Read the model definition and answer for the solid it produces. Units are mm, in the model's axes. Round coordinates to 2 decimals unless told otherwise and drop trailing zeros. Use a Markdown table: item, result. Add a question column.
1. The mould has two halves that part along X. Classify faces 1 (the face through (96, 0.5, -2)), 2 (the face through (52.3, 0.2, 13.6)), 3 (the face through (42.69, 0.25, -6.85)): +X half, -X half, draft (parallel to the pull), parting line (faces both ways), or undercut.
2. Section A-A, the plane y = 0.35 is taken. Give the number of separate pieces and of enclosed holes in the cut face, then the cut area to 3 significant figures.
3. Consider L1, parallel to Z at x = 58, y = 0.4; L2, parallel to Z at x = 27, y = 0.2. Determine where each line is inside the solid, lowest interval first. Write a range as [from, to].
```python
from build123d import *

# Parameters (mm, degrees)
SKETCH1_W           = 192.336493245
SKETCH1_H           = 38.107536872
BOSS_EXTRUDE1_DEPTH = 0.5


with BuildPart() as part:
    # Sketch1 → Boss-Extrude1 (new body)
    with BuildSketch(Plane(origin=(0, 0, 0), x_dir=(1, 0, 0), z_dir=(0, 1, 0))):
        with Locations((76.086163536, 1.75)):
            Rectangle(SKETCH1_W, SKETCH1_H)
        with BuildLine():
            Line((-17.791271396, 9.694580127), (-8.803798051, 0.707106781))
            ThreePointArc((-8.803798051, 0.707106781), (-7.096691269, 0), (-8.803798051, -0.707106781))
            Line((-8.803798051, -0.707106781), (-17.791271396, -9.694580127))
            ThreePointArc((-17.791271396, -9.694580127), (-17.791271396, -13.512956745), (-13.972894778, -13.512956745))
            Line((-13.972894778, -13.512956745), (-0.459938033, 0))
            Line((-0.459938033, 0), (-13.972894778, 13.512956745))
            ThreePointArc((-13.972894778, 13.512956745), (-17.791271396, 13.512956745), (-17.791271396, 9.694580127))
        make_face(mode=Mode.SUBTRACT)
        with BuildLine():
            Line((-3.972894778, 13.512956745), (9.540061967, 0))
            Line((9.540061967, 0), (-3.972894778, -13.512956745))
            ThreePointArc((-3.972894778, -13.512956745), (-7.791271396, -13.512956745), (-7.791271396, -9.694580127))
            Line((-7.791271396, -9.694580127), (1.196201949, -0.707106781))
            ThreePointArc((1.196201949, -0.707106781), (2.903308731, 0), (1.196201949, 0.707106781))
            Line((1.196201949, 0.707106781), (-7.791271396, 9.694580127))
            ThreePointArc((-7.791271396, 9.694580127), (-7.791271396, 13.512956745), (-3.972894778, 13.512956745))
        make_face(mode=Mode.SUBTRACT)
        with BuildLine():
            Line((6.027105222, 13.512956745), (19.540061967, 0))
            Line((19.540061967, 0), (6.027105222, -13.512956745))
            ThreePointArc((6.027105222, -13.512956745), (2.208728604, -13.512956745), (2.208728604, -9.694580127))
            Line((2.208728604, -9.694580127), (11.196201949, -0.707106781))
            ThreePointArc((11.196201949, -0.707106781), (12.903308731, 0), (11.196201949, 0.707106781))
            Line((11.196201949, 0.707106781), (2.208728604, 9.694580127))
            ThreePointArc((2.208728604, 9.694580127), (2.208728604, 13.512956745), (6.027105222, 13.512956745))
        make_face(mode=Mode.SUBTRACT)
        with BuildLine():
            Line((16.027105222, 13.512956745), (29.540061967, 0))
            Line((29.540061967, 0), (16.027105222, -13.512956745))
            ThreePointArc((16.027105222, -13.512956745), (12.208728604, -13.512956745), (12.208728604, -9.694580127))
            Line((12.208728604, -9.694580127), (21.196201949, -0.707106781))
            ThreePointArc((21.196201949, -0.707106781), (22.903308731, 0), (21.196201949, 0.707106781))
            Line((21.196201949, 0.707106781), (12.208728604, 9.694580127))
            ThreePointArc((12.208728604, 9.694580127), (12.208728604, 13.512956745), (16.027105222, 13.512956745))
        make_face(mode=Mode.SUBTRACT)
        with BuildLine():
            Line((26.027105222, 13.512956745), (39.540061967, 0))
            Line((39.540061967, 0), (26.027105222, -13.512956745))
            ThreePointArc((26.027105222, -13.512956745), (22.208728604, -13.512956745), (22.208728604, -9.694580127))
            Line((22.208728604, -9.694580127), (31.196201949, -0.707106781))
            ThreePointArc((31.196201949, -0.707106781), (32.903308731, 0), (31.196201949, 0.707106781))
            Line((31.196201949, 0.707106781), (22.208728604, 9.694580127))
            ThreePointArc((22.208728604, 9.694580127), (22.208728604, 13.512956745), (26.027105222, 13.512956745))
        make_face(mode=Mode.SUBTRACT)
        with BuildLine():
            Line((36.027105222, 13.512956745), (49.540061967, 0))
            Line((49.540061967, 0), (36.027105222, -13.512956745))
            ThreePointArc((36.027105222, -13.512956745), (32.208728604, -13.512956745), (32.208728604, -9.694580127))
            Line((32.208728604, -9.694580127), (41.196201949, -0.707106781))
            ThreePointArc((41.196201949, -0.707106781), (42.903308731, 0), (41.196201949, 0.707106781))
            Line((41.196201949, 0.707106781), (32.208728604, 9.694580127))
            ThreePointArc((32.208728604, 9.694580127), (32.208728604, 13.512956745), (36.027105222, 13.512956745))
        make_face(mode=Mode.SUBTRACT)
        with BuildLine():
            Line((46.027105222, 13.512956745), (59.540061967, 0))
            Line((59.540061967, 0), (46.027105222, -13.512956745))
            ThreePointArc((46.027105222, -13.512956745), (42.208728604, -13.512956745), (42.208728604, -9.694580127))
            Line((42.208728604, -9.694580127), (51.196201949, -0.707106781))
            ThreePointArc((51.196201949, -0.707106781), (52.903308731, 0), (51.196201949, 0.707106781))
            Line((51.196201949, 0.707106781), (42.208728604, 9.694580127))
            ThreePointArc((42.208728604, 9.694580127), (42.208728604, 13.512956745), (46.027105222, 13.512956745))
        make_face(mode=Mode.SUBTRACT)
        with BuildLine():
            Line((56.027105222, 13.512956745), (69.540061967, 0))
            Line((69.540061967, 0), (56.027105222, -13.512956745))
            ThreePointArc((56.027105222, -13.512956745), (52.208728604, -13.512956745), (52.208728604, -9.694580127))
            Line((52.208728604, -9.694580127), (61.196201949, -0.707106781))
            ThreePointArc((61.196201949, -0.707106781), (62.903308731, 0), (61.196201949, 0.707106781))
            Line((61.196201949, 0.707106781), (52.208728604, 9.694580127))
            ThreePointArc((52.208728604, 9.694580127), (52.208728604, 13.512956745), (56.027105222, 13.512956745))
        make_face(mode=Mode.SUBTRACT)
        with BuildLine():
            Line((66.027105222, 13.512956745), (79.540061967, 0))
            Line((79.540061967, 0), (66.027105222, -13.512956745))
            ThreePointArc((66.027105222, -13.512956745), (62.208728604, -13.512956745), (62.208728604, -9.694580127))
            Line((62.208728604, -9.694580127), (71.196201949, -0.707106781))
            ThreePointArc((71.196201949, -0.707106781), (72.903308731, 0), (71.196201949, 0.707106781))
            Line((71.196201949, 0.707106781), (62.208728604, 9.694580127))
            ThreePointArc((62.208728604, 9.694580127), (62.208728604, 13.512956745), (66.027105222, 13.512956745))
        make_face(mode=Mode.SUBTRACT)
        with BuildLine():
            Line((76.027105222, 13.512956745), (89.540061967, 0))
            Line((89.540061967, 0), (76.027105222, -13.512956745))
            ThreePointArc((76.027105222, -13.512956745), (72.208728604, -13.512956745), (72.208728604, -9.694580127))
            Line((72.208728604, -9.694580127), (81.196201949, -0.707106781))
            ThreePointArc((81.196201949, -0.707106781), (82.903308731, 0), (81.196201949, 0.707106781))
            Line((81.196201949, 0.707106781), (72.208728604, 9.694580127))
            ThreePointArc((72.208728604, 9.694580127), (72.208728604, 13.512956745), (76.027105222, 13.512956745))
        make_face(mode=Mode.SUBTRACT)
    extrude(amount=BOSS_EXTRUDE1_DEPTH)


solid = part.part
```
Verdict:
| question | item | result |
|---|---|---|
| 1 | face 1 | draft |
| 1 | face 2 | undercut |
| 1 | face 3 | undercut |
| 2 | separate pieces | 1 |
| 2 | enclosed holes | 10 |
| 2 | area | 5,350 mm2 |
| 3 | L1 | z = [-20.8, -11.54], [-3.9, -1.54], [1.54, 3.9], [11.54, 17.3] |
| 3 | L2 | z = [-20.8, -12.54], [-4.9, -2.54], [2.54, 4.9], [12.54, 17.3] |
